from build123d import *

# Parameters (mm, degrees)
SKETCH_1_W                    = 27.2
SKETCH_1_H                    = 27.2
EXTRUDE_480_DEPTH             = 1.2
SKETCH_2_W                    = 27.2
SKETCH_2_H                    = 19.26
EXTRUDE_643_DEPTH             = 1.8
EXTRUDE_867_REACH             = 21.317
SKETCH_3_R                    = 0.5
EXTRUDE_867_DIRECTION_2_DEPTH = 9.2
SKETCH_4_R                    = 1.5
CUT_EXTRUDE_1140_DEPTH        = 22.320412754
SKETCH_5_W                    = 10.16
SKETCH_5_H                    = 2.54
EXTRUDE_1389_DEPTH            = 2
SKETCH_7_W                    = 10.16
SKETCH_7_H                    = 2.54
EXTRUDE_2113_DEPTH            = 17


with BuildPart() as part:
    # Эскиз1 → Extrude 480 (new body)
    with BuildSketch(Plane.XY):
        Rectangle(SKETCH_1_W, SKETCH_1_H)
    extrude(amount=EXTRUDE_480_DEPTH)

    # Эскиз2 → Extrude 643 (add)
    with BuildSketch(Plane.XY.offset(1.2)):
        Rectangle(SKETCH_2_W, SKETCH_2_H)
    extrude(amount=EXTRUDE_643_DEPTH)

    # Extrude 867: up to this face of the body (flat: up to its plane)
    extrude_867_end = Plane(part.part.faces().sort_by_distance((0, 0, 3))[0])
    # Эскиз3 → Extrude 867 (add, up to the picked face)
    with BuildSketch(Plane.XY.offset(1.2), mode=Mode.PRIVATE) as extrude_867_sk1:
        with Locations((-3.81, 12.1)):
            Circle(SKETCH_3_R)
    extrude_867_tool1 = split(extrude(extrude_867_sk1.sketch, amount=EXTRUDE_867_REACH, mode=Mode.PRIVATE), bisect_by=extrude_867_end, keep=Keep.BOTH, mode=Mode.PRIVATE)
    # Эскиз3 → Extrude 867 (add, up to the picked face)
    with BuildSketch(Plane.XY.offset(1.2), mode=Mode.PRIVATE) as extrude_867_sk2:
        with Locations((-1.27, 12.1)):
            Circle(SKETCH_3_R)
    extrude_867_tool2 = split(extrude(extrude_867_sk2.sketch, amount=EXTRUDE_867_REACH, mode=Mode.PRIVATE), bisect_by=extrude_867_end, keep=Keep.BOTH, mode=Mode.PRIVATE)
    # Эскиз3 → Extrude 867 (add, up to the picked face)
    with BuildSketch(Plane.XY.offset(1.2), mode=Mode.PRIVATE) as extrude_867_sk3:
        with Locations((1.27, 12.1)):
            Circle(SKETCH_3_R)
    extrude_867_tool3 = split(extrude(extrude_867_sk3.sketch, amount=EXTRUDE_867_REACH, mode=Mode.PRIVATE), bisect_by=extrude_867_end, keep=Keep.BOTH, mode=Mode.PRIVATE)
    # Эскиз3 → Extrude 867 (add, up to the picked face)
    with BuildSketch(Plane.XY.offset(1.2), mode=Mode.PRIVATE) as extrude_867_sk4:
        with Locations((3.81, 12.1)):
            Circle(SKETCH_3_R)
    extrude_867_tool4 = split(extrude(extrude_867_sk4.sketch, amount=EXTRUDE_867_REACH, mode=Mode.PRIVATE), bisect_by=extrude_867_end, keep=Keep.BOTH, mode=Mode.PRIVATE)
    add(extrude_867_tool1.solids().sort_by(Axis((-3.81, 12.1, 1.2), (0, 0, 1)))[0])
    add(extrude_867_tool2.solids().sort_by(Axis((-1.27, 12.1, 1.2), (0, 0, 1)))[0])
    add(extrude_867_tool3.solids().sort_by(Axis((1.27, 12.1, 1.2), (0, 0, 1)))[0])
    add(extrude_867_tool4.solids().sort_by(Axis((3.81, 12.1, 1.2), (0, 0, 1)))[0])

    # Эскиз3 → Extrude 867 direction 2 (add)
    with BuildSketch(Plane.XY.offset(1.2)):
        with Locations((-3.81, 12.1)):
            Circle(SKETCH_3_R)
        with Locations((-1.27, 12.1)):
            Circle(SKETCH_3_R)
        with Locations((1.27, 12.1)):
            Circle(SKETCH_3_R)
        with Locations((3.81, 12.1)):
            Circle(SKETCH_3_R)
    extrude(amount=-EXTRUDE_867_DIRECTION_2_DEPTH)

    # Эскиз4 → Cut-Extrude 1140 (cut, through all)
    with BuildSketch(Plane.XY.offset(1.2)):
        with Locations((-11.6, 11.6)):
            Circle(SKETCH_4_R)
        with Locations((11.6, 11.6)):
            Circle(SKETCH_4_R)
        with Locations((11.6, -11.6)):
            Circle(SKETCH_4_R)
        with Locations((-11.6, -11.6)):
            Circle(SKETCH_4_R)
    extrude(amount=-CUT_EXTRUDE_1140_DEPTH, mode=Mode.SUBTRACT)

    # Эскиз5 → Extrude 1389 (add)
    with BuildSketch(Plane(origin=(0, 0, 0), x_dir=(-1, 0, 0), z_dir=(0, 0, -1))):
        with Locations((0, 12.1)):
            Rectangle(SKETCH_5_W, SKETCH_5_H)
    extrude(amount=EXTRUDE_1389_DEPTH)

    # Эскиз7 → Extrude 2113 (add)
    with BuildSketch(Plane(origin=(0, 0, -2), x_dir=(-1, 0, 0), z_dir=(0, 0, -1))):
        with Locations((0, 12.1)):
            Rectangle(SKETCH_7_W, SKETCH_7_H)
    extrude(amount=EXTRUDE_2113_DEPTH)


solid = part.part
Source: CAD feature listing. Evaluate the final solid. Frame: model axes, mm. A direction names the side the tool comes from. Coordinates: 2 decimals unless noted, no trailing zeros. Loops run counter-clockwise (first coordinate to the right, second up) from the corner with the lowest first, then second, coordinate; pieces in that order, holes last. Notation, with made-up numbers: (58.25, 27.5) - (67.25, 27.5) arc R21 cw to (67.25, 50.5) - close; hole circle Ø8 at (88, 21). An arc over 180 degrees is marked (long way). One line per item, written item: value. Start each with the question number.
1. Section B-B (y = -11.6). Return the cut outline in (x, z).
2. Contact query for flat-ended pins moving along their axis: P1, Ø5, axis at x = -1, z = -10.5, coming from the +Y side; P2, Ø1.3, axis at y = 12, z = -10, coming from the -X side; P3, Ø2, axis at y = 12, z = -13, coming from the +X side; P4, Ø2, axis at x = -7.5, z = -5.5, coming from the -Y side. Output: stop coordinate, or through.
3. Section A-A (x = 11.6). Return the cut outline in (y, z), and give its area (3 significant figures).
4. Set-up query: faces 1 (the flat face through (5.08, 12, -9)), 2 (the cylindrical face through (1.501, 11.656, 2.087)), 3 (the flat face through (0, 13.37, -9)), 4 (the flat face through (0, 10.83, -9)), 5 (the flat face through (0, -12, 1.2)). Return all of +Z, -Z, +X, -X, +Y, -Y with unobstructed straight access to the full face (end or side cutting, diameter ignored); none if empty.
5. Ray query, L1, parallel to Y at x = 11.6, z = 0.95; L2, parallel to Z at x = -3.75, y = 3.25; L3, parallel to Y at x = 2, z = -12.75. Return the intervals inside material, ascending.
6. Mould query, pull axis X, two halves, no side actions, for faces 6 (the cylindrical face through (-13.1, -11.53, 0.61)), 7 (the flat face through (0, 12, -19)), 8 (the flat face through (13.6, 0, 1)). Classes: pulls with the +X half, pulls with the -X half, needs draft (parallel to the pull), parting line crosses it, or undercut.
7. Section C-C (x = 1.27). Return the cut outline in (y, z).
8. Section D-D (y = 12.1). State how many separate pieces and enclosed holes the cut face has, and give its area (3 significant figures).
Verdict:
1. outline: (-13.6, 0) - (-13.1, 0) - (-13.1, 1.2) - (-13.6, 1.2) - close; (-10.1, 0) - (10.1, 0) - (10.1, 1.2) - (-10.1, 1.2) - close; (13.1, 0) - (13.6, 0) - (13.6, 1.2) - (13.1, 1.2) - close
2. P1: stops at y = 13.37
2. P2: stops at x = -5.08
2. P3: stops at x = 5.08
2. P4: passes through
3. outline: (-13.6, 0) - (-13.1, 0) - (-13.1, 1.2) - (-13.6, 1.2) - close; (-10.1, 0) - (10.1, 0) - (10.1, 1.2) - (9.63, 1.2) - (9.63, 3) - (-9.63, 3) - (-9.63, 1.2) - (-10.1, 1.2) - close; (13.1, 0) - (13.6, 0) - (13.6, 1.2) - (13.1, 1.2) - close
3. area: 60.1 mm2
4. face 1: -Z, +X, +Y, -Y
4. face 2: +Z
4. face 3: -Z, +X, -X, +Y
4. face 4: -Z, +X, -X, -Y
4. face 5: +Z, +X, -X, -Y
5. L1: y = -13.6 to -13.1, -10.1 to 10.1, 13.1 to 13.6
5. L2: z = 0 to 3
5. L3: y = 10.83 to 13.37
6. face 6: undercut
6. face 7: needs draft
6. face 8: pulls with the +X half
7. outline: (-13.6, 0) - (10.83, 0) - (10.83, -19) - (13.37, -19) - (13.37, 0) - (13.6, 0) - (13.6, 1.2) - (12.6, 1.2) - (12.6, 3) - (11.6, 3) - (11.6, 1.2) - (9.63, 1.2) - (9.63, 3) - (-9.63, 3) - (-9.63, 1.2) - (-13.6, 1.2) - close
8. separate pieces: 3
8. enclosed holes: 0
8. area: 226 mm2
